The listing builds one solid part. Answer for the finished solid, in the listing's coordinates (mm). Coordinates: 2 decimals unless noted, no trailing zeros. Order: outer loops, then holes, each group sorted by start corner. A loop starts at its lowest first (then second) coordinate and runs counter-clockwise, first axis right, second up. Notation, with made-up numbers: (59, 60) -> (77, 60) arc R24 ccw to (77, 89) -> close; hole circle Ø8 at (-32, 84.5). An arc over 180 degrees is marked (long way). Return JSON: item names as keys, results as strings.
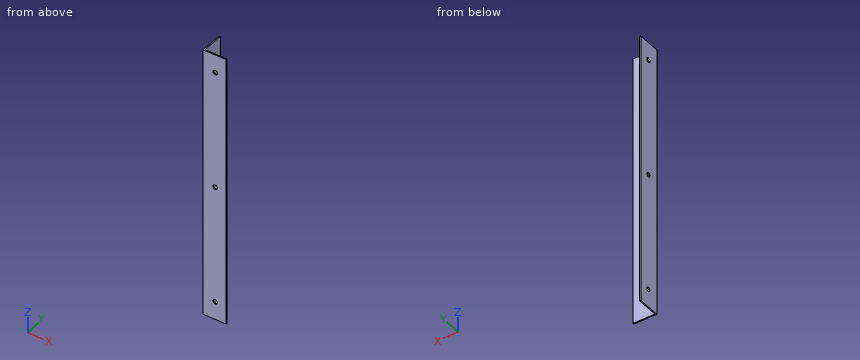
Autodesk Inventor part; units mm, degrees
ref_plane "YZ Plane" through (0, 0, 0) normal (1, 0, 0) x (0, 1, 0)
ref_plane "XZ Plane" through (0, 0, 0) normal (0, 1, 0) x (-1, 0, 0)
ref_plane "XY Plane" through (0, 0, 0) normal (0, 0, 1) x (1, 0, 0)
sketch "Sketch1" plane through (0, 0, 0) normal (0, 0, 1) x (1, 0, 0)
  line L0 (0, 0) -> (0, 15.875)
  line L1 (0, 15.875) -> (0.7937, 15.875)
  line L2 (0.7937, 15.875) -> (0.7938, 0.7937)
  line L3 (0.7938, 0.7937) -> (15.875, 0.7937)
  line L4 (15.875, 0.7937) -> (15.875, 0)
  line L5 (15.875, 0) -> (0, 0)
  dimension "d0" = 15.875
  dimension "d1" = 0.7937
extrude "Extrusion1" add sketch "Sketch1" along normal blind 190.5
sketch "Sketch2" plane through (0.7938, 0.7937, 0) normal (0, 1, 0) x (1, 0, 0)
  line L0 (0, 0) -> (15.0812, 0)
  line L1 (15.0812, -190.5) -> (0, -190.5)
  line L2 (7.5406, 0) -> (7.5406, -190.5) construction
  circle A0 centre (7.5406, -12.7) radius 1.5875
  circle A1 centre (7.5406, -95.25) radius 1.5875
  circle A2 centre (7.5406, -177.8) radius 1.5875
  point P0 (-0.7938, 0)
  dimension "d4" = 12.7
  dimension "d5" = 3.175
  dimension "d6" = 190.5
  dimension "d9" = 82.55
sketch "Sketch3" plane through (0.7938, 0.7937, 0) normal (1, 0, 0) x (0, 0, -1)
  line L0 (0, 15.0812) -> (0, 0)
  line L1 (-190.5, 0) -> (-190.5, 15.0812)
  line L2 (-190.5, 7.5406) -> (0, 7.5406) construction
  circle A0 centre (-12.7, 7.5406) radius 1.5875
  circle A1 centre (-95.25, 7.5406) radius 1.5875
  circle A2 centre (-177.8, 7.5406) radius 1.5875
  point P0 (0, -0.7937)
  dimension "d14" = 3.175
  dimension "d15" = 12.7
  dimension "d16" = 190.5
  dimension "d19" = 82.55
extrude "Extrusion2" cut sketch "Sketch2" against normal through all
extrude "Extrusion3" cut sketch "Sketch3" against normal through all
properties part number "Hopper Bracing Front Left P5" material "Aluminum 6061"
1. Consider line 1 (X direction, y = 0.2, z = 12.7) (3 decimals); line 2 (X direction, y = 9.5, z = 98). Determine where each line is inside the solid, lowest interval first. Write a range as from..to.
Answer block:
{"line 1": "x = 0..6.747, 9.922..15.875", "line 2": "x = 0..0.79"}
2. The part is cut by section A-A on z = 95.25. Give the vertices of the cut face in (x, y) (3 decimals), and give its area (3 significant figures).
Answer block:
{"outline": "(0, 0) -> (6.747, 0) -> (6.747, 0.794) -> (0.794, 0.794) -> (0.794, 6.747) -> (0, 6.747) -> close; (0, 9.922) -> (0.794, 9.922) -> (0.794, 15.875) -> (0, 15.875) -> close; (9.922, 0) -> (15.875, 0) -> (15.875, 0.794) -> (9.922, 0.794) -> close", "area": "19.5 mm2"}
3. Each of these flat-tipped pins is pushed along its axis until it touches: pin 1 Ø5 at (y, z) = (3.5, 34.5) entering from +X; pin 2 Ø4 at (x, z) = (8.33, 177.8) entering from +Y. Where does it stop, or does it pass through?
Answer block:
{"pin 1": "stops at x = 0.79", "pin 2": "stops at y = 0.79"}
4. The part is cut by section B-B on x = 12. Give the vertices of the cut face in (y, z).
Answer block:
{"outline": "(0, 0) -> (0.79, 0) -> (0.79, 190.5) -> (0, 190.5) -> close"}
